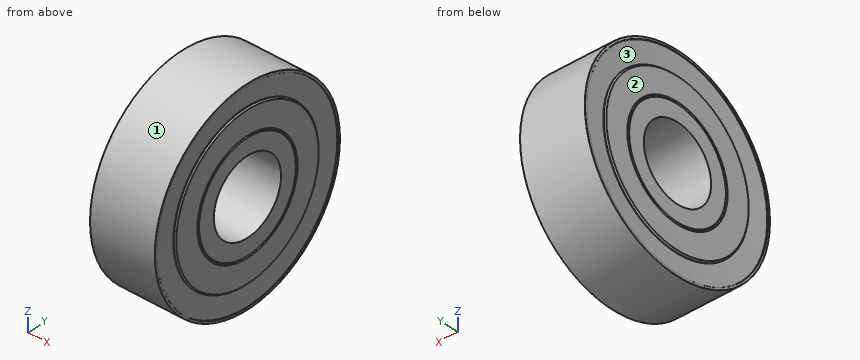
```python
from build123d import *


with BuildPart() as part:
    # Sketch1 → Revolve1 (revolve)
    with BuildSketch(Plane.XY):
        Polygon((-3.5, 4), (3.5, 4), (3.5, 5.75), (3.393933983, 5.856066017), (3.5, 5.962132034), (3.5, 8.462132034), (3.358578644, 8.603553391), (3.308578644, 8.603553391), (3.429289322, 10.75), (3.49, 10.75), (3.5, 10.76), (3.5, 10.99), (3.489185937, 11), (-3.489185937, 11), (-3.5, 10.99), (-3.5, 10.76), (-3.49, 10.75), (-3.429289322, 10.75), (-3.308578644, 8.603553391), (-3.358578644, 8.603553391), (-3.5, 8.462132034), (-3.5, 5.962132034), (-3.393933983, 5.856066017), (-3.5, 5.75), align=None)
    revolve(axis=Axis((-0.54284752, 0, 0), (1, 0, 0)))


solid = part.part
```
CAD build for the part. Positions are in the model's coordinates, mm. Face numbers are marked on the shaded views. Give positions to 0.01 mm unless a question says otherwise; leave off trailing zeros. Order: outer loops, then holes, each group sorted by start corner. A loop starts at its lowest first (then second) coordinate and runs counter-clockwise, first axis right, second up. Notation, with made-up numbers: M 11,13 L 56,13 A15 cw 56,32 Z; hole C 45.5,-37 d11. An arc over 180 degrees is marked long. Put each result on its own line as item: value. Start each with the question number.
(1) Flat gauge pins, fed straight in: pin 1 Ø1.5 at (x, z) = (2, 4) entering from -Y; pin 2 Ø2 at (x, y) = (-0.5, -8.5) entering from -Z; pin 3 Ø10.5 at (y, z) = (0, 0) entering from -X; pin 4 Ø2 at (x, y) = (1.5, -5) entering from +Z. Where does each tip first touch, or does it go through?
(2) Drill centre lines: line 1 along Z through (x, y) = (-1.5, 0); line 2 along Z through (x, y) = (-0.5, -1.5); line 3 along X through (y, z) = (9, -2.75). Where is each one in solid material? Low to high.
(3) Saw through at A-A, the plane x = -0.25. Write the cut outline in (y, z), then the cut area to 3 significant figures.
(4) Mould opens along Y. For the marked faces 1, 2 and 3 say: +Y half, -Y half, draft (parallel to the pull), parting line (faces both ways), or undercut.
Check result:
1. pin 1: stops at y = -10.51
1. pin 2: stops at z = -8.05
1. pin 3: stops at x = -3.5
1. pin 4: stops at z = 10.25
2. line 1: z = -11 to -4, 4 to 11
2. line 2: z = -10.9 to -3.71, 3.71 to 10.9
2. line 3: x = -3.35 to 3.35
3. outline: C 0,0 d22; hole C 0,0 d8
3. area: 330 mm2
4. face 1: parting line
4. face 2: draft
4. face 3: undercut
